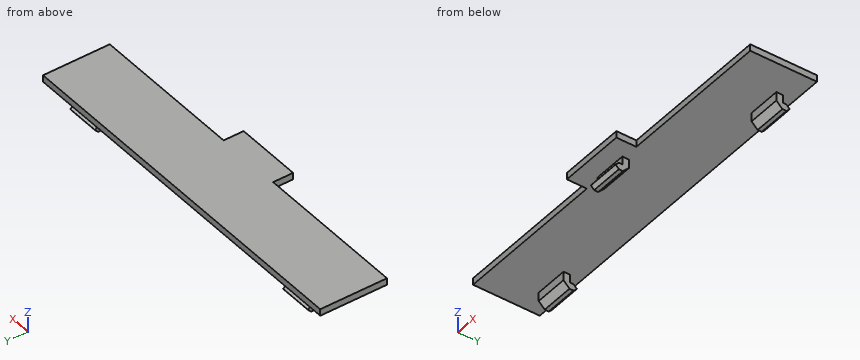
from build123d import *

# Parameters (mm, degrees)
BOX082_W                  = 56
BOX082_H                  = 10
BOX082_DEPTH              = 1
BOX081_W                  = 10
BOX081_H                  = 10
BOX081_DEPTH              = 1
BOX085_W                  = 5
BOX085_H                  = 1
BOX085_DEPTH              = 1
CHAMFER013_SIZE           = 0.49
BOX086_W                  = 5
BOX086_H                  = 1
BOX086_DEPTH              = 2.2
CHAMFER014_SIZE           = 0.9
FUSION078_PLACEMENT_ANGLE = 180
BOX088_W                  = 5
BOX088_H                  = 1
BOX088_DEPTH              = 1
CHAMFER015_SIZE           = 0.49
BOX087_W                  = 5
BOX087_H                  = 1
BOX087_DEPTH              = 2.2
CHAMFER016_SIZE           = 0.9
FUSION079_PLACEMENT_ANGLE = 180
BOX083_W                  = 5
BOX083_H                  = 1
BOX083_DEPTH              = 1
CHAMFER011_SIZE           = 0.49
BOX084_W                  = 5
BOX084_H                  = 1
BOX084_DEPTH              = 2.2
CHAMFER012_SIZE           = 0.9


with BuildPart() as obj1:
    # Box082 → Box082 (new body)
    with BuildSketch(Plane(origin=(-38, 19.5, 14.75), x_dir=(1, 0, 0), z_dir=(0, 0, 1))):
        with Locations((28, 5)):
            Rectangle(BOX082_W, BOX082_H)
    extrude(amount=BOX082_DEPTH)


with BuildPart() as obj2:
    # Box081 → Box081 (new body)
    with BuildSketch(Plane(origin=(-15, 16.5, 14.75), x_dir=(1, 0, 0), z_dir=(0, 0, 1))):
        with Locations((5, 5)):
            Rectangle(BOX081_W, BOX081_H)
    extrude(amount=BOX081_DEPTH)

    # Fusion077: union obj1
    add(obj1.part)


with BuildPart() as chamfer013:
    # Box085 → Box085 (new body)
    with BuildSketch(Plane(origin=(-12.5, 18.25, 12.75), x_dir=(1, 0, 0), z_dir=(0, 0, 1))):
        with Locations((2.5, 0.5)):
            Rectangle(BOX085_W, BOX085_H)
    extrude(amount=BOX085_DEPTH)

    # Chamfer013
    chamfer013_edges = [chamfer013.edges().sort_by_distance(p)[0] for p in [
        (-10, 18.25, 12.75),
        (-10, 18.25, 13.75),
    ]]
    chamfer(chamfer013_edges, length=CHAMFER013_SIZE)


with BuildPart() as chamfer013_1:
    # Chamfer013 placement: moved
    add(chamfer013.part.moved(Location((0, 0, -0.2))))


with BuildPart() as obj3:
    # Box086 → Box086 (new body)
    with BuildSketch(Plane(origin=(-12.5, 19.25, 12.55), x_dir=(1, 0, 0), z_dir=(0, 0, 1))):
        with Locations((2.5, 0.5)):
            Rectangle(BOX086_W, BOX086_H)
    extrude(amount=BOX086_DEPTH)

    # Chamfer014
    chamfer014_edges = [obj3.edges().sort_by_distance(p)[0] for p in [
        (-10, 20.25, 12.55),
    ]]
    chamfer(chamfer014_edges, length=CHAMFER014_SIZE)

    # Fusion078: union Chamfer013
    add(chamfer013_1.part)


with BuildPart() as obj3_1:
    # Fusion078 placement: moved
    add(obj3.part.moved(Location((1, 47, 0))).rotate(Axis((1, 47, 0), (0, 0, 1)), FUSION078_PLACEMENT_ANGLE))


with BuildPart() as chamfer015:
    # Box088 → Box088 (new body)
    with BuildSketch(Plane(origin=(-12.5, 18.25, 12.75), x_dir=(1, 0, 0), z_dir=(0, 0, 1))):
        with Locations((2.5, 0.5)):
            Rectangle(BOX088_W, BOX088_H)
    extrude(amount=BOX088_DEPTH)

    # Chamfer015
    chamfer015_edges = [chamfer015.edges().sort_by_distance(p)[0] for p in [
        (-10, 18.25, 12.75),
        (-10, 18.25, 13.75),
    ]]
    chamfer(chamfer015_edges, length=CHAMFER015_SIZE)


with BuildPart() as chamfer015_1:
    # Chamfer015 placement: moved
    add(chamfer015.part.moved(Location((0, 0, -0.2))))


with BuildPart() as obj4:
    # Box087 → Box087 (new body)
    with BuildSketch(Plane(origin=(-12.5, 19.25, 12.55), x_dir=(1, 0, 0), z_dir=(0, 0, 1))):
        with Locations((2.5, 0.5)):
            Rectangle(BOX087_W, BOX087_H)
    extrude(amount=BOX087_DEPTH)

    # Chamfer016
    chamfer016_edges = [obj4.edges().sort_by_distance(p)[0] for p in [
        (-10, 20.25, 12.55),
    ]]
    chamfer(chamfer016_edges, length=CHAMFER016_SIZE)

    # Fusion079: union Chamfer015
    add(chamfer015_1.part)


with BuildPart() as obj4_1:
    # Fusion079 placement: moved
    add(obj4.part.moved(Location((-42, 47, 0))).rotate(Axis((-42, 47, 0), (0, 0, 1)), FUSION079_PLACEMENT_ANGLE))


with BuildPart() as chamfer011:
    # Box083 → Box083 (new body)
    with BuildSketch(Plane(origin=(-12.5, 18.25, 12.75), x_dir=(1, 0, 0), z_dir=(0, 0, 1))):
        with Locations((2.5, 0.5)):
            Rectangle(BOX083_W, BOX083_H)
    extrude(amount=BOX083_DEPTH)

    # Chamfer011
    chamfer011_edges = [chamfer011.edges().sort_by_distance(p)[0] for p in [
        (-10, 18.25, 12.75),
        (-10, 18.25, 13.75),
    ]]
    chamfer(chamfer011_edges, length=CHAMFER011_SIZE)


with BuildPart() as chamfer011_1:
    # Chamfer011 placement: moved
    add(chamfer011.part.moved(Location((0, 0, -0.2))))


with BuildPart() as abdeckung_gpio:
    # Box084 → Box084 (new body)
    with BuildSketch(Plane(origin=(-12.5, 19.25, 12.55), x_dir=(1, 0, 0), z_dir=(0, 0, 1))):
        with Locations((2.5, 0.5)):
            Rectangle(BOX084_W, BOX084_H)
    extrude(amount=BOX084_DEPTH)

    # Chamfer012
    chamfer012_edges = [abdeckung_gpio.edges().sort_by_distance(p)[0] for p in [
        (-10, 20.25, 12.55),
    ]]
    chamfer(chamfer012_edges, length=CHAMFER012_SIZE)

    # Fusion076: union Chamfer011
    add(chamfer011_1.part)

    # Fusion080: union obj3, obj4
    add(obj3_1.part)
    add(obj4_1.part)

    # Fusion081: union obj2
    add(obj2.part)


solid = abdeckung_gpio.part
Here's how the part is built. I have some questions about the finished solid (model axes, mm). Round coordinates to 2 decimals unless told otherwise and drop trailing zeros. Write each loop counter-clockwise with the first axis right and the second up, starting at its lowest first coordinate (ties: lowest second). Pieces come first, ordered by that corner, then holes.
1. I need wall thicknesses on L1, parallel to X at y = 28, z = 12.9; L2, parallel to Z at x = -2.5, y = 23.75; L3, parallel to Y at x = 1, z = 15. Which ranges of each line are inside material? Lowest first, please.
2. Suppose I cut it at C-C (y = 26.25). List the corners of the cut face in (x, z) for me.
3. Will these pins go through, and if not, where does the flat tip stop? pin 1 Ø1.1 at (y, z) = (17.5, 15) entering from -X; pin 2 Ø1 at (y, z) = (27.5, 14) entering from +X; pin 3 Ø1 at (y, z) = (19.5, 13) entering from -X.
4. Suppose I cut it at D-D (y = 17.75). List the corners of the cut face in (x, z) for me.
Answer sheet:
1. L1: x = -34.5 to -29.5, 8.5 to 13.5
1. L2: z = 14.75 to 15.75
1. L3: y = 19.5 to 29.5
2. outline: (-38, 14.75) - (18, 14.75) - (18, 15.75) - (-38, 15.75) - close
3. pin 1: stops at x = -15
3. pin 2: stops at x = 13.5
3. pin 3: stops at x = -12.5
4. outline: (-15, 14.75) - (-5, 14.75) - (-5, 15.75) - (-15, 15.75) - close
